```python
from build123d import *

# Parameters (mm, degrees)
SKETCH_W        = 76
SKETCH_H        = 22
PAD_DEPTH       = 76
SKETCH001_W     = 66
SKETCH001_H     = 26
PAD001_DEPTH    = 32
SKETCH002_W     = 62
SKETCH002_H     = 22
POCKET_DEPTH    = 30
SKETCH003_W     = 72
SKETCH003_H     = 18
POCKET001_DEPTH = 74
SKETCH004_W     = 30
SKETCH004_H     = 2
POCKET002_DEPTH = 30
SKETCH005_W     = 30
SKETCH005_H     = 2
POCKET003_DEPTH = 74


with BuildPart() as part:
    # Sketch → Pad (new body)
    with BuildSketch(Plane.XY):
        with Locations((38, 11)):
            Rectangle(SKETCH_W, SKETCH_H)
    extrude(amount=PAD_DEPTH)

    # Sketch001 → Pad001 (join)
    with BuildSketch(Plane.XY):
        with Locations((38, -13)):
            Rectangle(SKETCH001_W, SKETCH001_H)
    extrude(amount=PAD001_DEPTH)

    # Sketch002 (on Face4 of Pad001) → Pocket (cut)
    with BuildSketch(Plane.XY.offset(32)):
        with Locations((38, -13)):
            Rectangle(SKETCH002_W, SKETCH002_H)
    extrude(amount=-POCKET_DEPTH, mode=Mode.SUBTRACT)

    # Sketch003 (on Face7 of Pocket) → Pocket001 (cut)
    with BuildSketch(Plane.XY.offset(76)):
        with Locations((38, 11)):
            Rectangle(SKETCH003_W, SKETCH003_H)
    extrude(amount=-POCKET001_DEPTH, mode=Mode.SUBTRACT)

    # Sketch004 (on Face4 of Pocket001) → Pocket002 (cut)
    with BuildSketch(Plane.XY.offset(32)):
        with Locations((38, -1)):
            Rectangle(SKETCH004_W, SKETCH004_H)
    extrude(amount=-POCKET002_DEPTH, mode=Mode.SUBTRACT)

    # Sketch005 (on Face8 of Pocket002) → Pocket003 (cut)
    with BuildSketch(Plane.XY.offset(76)):
        with Locations((38, 1)):
            Rectangle(SKETCH005_W, SKETCH005_H)
    extrude(amount=-POCKET003_DEPTH, mode=Mode.SUBTRACT)


solid = part.part
```
Work out the finished part from the listing and answer in its coordinate system (mm). A direction names the side the tool comes from. Coordinates: 2 decimals unless noted, no trailing zeros. Write each loop counter-clockwise with the first axis right and the second up, starting at its lowest first coordinate (ties: lowest second). Pieces come first, ordered by that corner, then holes.
Q1. A cutting plane is placed at A-A, the plane z = 15. Give the vertices of the cut face in (x, y).
Q2. A cutting plane is placed at D-D, the plane z = 47. Give the vertices of the cut face in (x, y), then the cut area to 3 significant figures.
Q3. Which of the six approach directions +Z, -Z, +X, -X, +Y, -Y give full straight-line access (tool end or side, diameter ignored) to faces 4 (the face through (37, 20, 40)), 5 (the face through (71, -13, 16)), 6 (the face through (37.8, -24.5, 32)), 7 (the face through (5, -13, 16))?
Q4. Find the intervals of material crossed by line 1 (Y direction, x = 18, z = 24); line 2 (X direction, y = 12.5, z = 6.5); line 3 (Y direction, x = 20, z = 65.5), in increasing order.
Q5. Each of these flat-tipped pins is pushed along its axis until it touches: pin 1 Ø11 at (y, z) = (-18, 15) entering from +X; pin 2 Ø1 at (x, y) = (8.5, -9.5) entering from +Z; pin 3 Ø11.5 at (x, z) = (67, 55) entering from -Y. Where does it stop, or does it pass through?
Q6. A cutting plane is placed at C-C, the plane x = 51. Give the vertices of the cut face in (y, z), then the cut area to 3 significant figures.
Q7. A cutting plane is placed at B-B, the plane y = 12. Give the vertices of the cut face in (x, z), then the cut area to 3 significant figures.
Q8. Determine the mould class of faces 1 (the face through (37, 22, 37)), 2 (the face through (37, -2, 0)), 3 (the face through (2, 11, 40)) for opening direction Y: released by +Y, released by -Y, zero draft, split by the parting line, or undercut.
Findings below:
1. outline: (0, 0) - (5, 0) - (5, -26) - (71, -26) - (71, 0) - (76, 0) - (76, 22) - (0, 22) - close; hole (2, 2) - (23, 2) - (23, -2) - (7, -2) - (7, -24) - (69, -24) - (69, -2) - (53, -2) - (53, 2) - (74, 2) - (74, 20) - (2, 20) - close
2. outline: (0, 0) - (23, 0) - (23, 2) - (2, 2) - (2, 20) - (74, 20) - (74, 2) - (53, 2) - (53, 0) - (76, 0) - (76, 22) - (0, 22) - close
2. area: 316 mm2
3. face 4: +Z
3. face 5: +Z, -Z, +X, -Y
3. face 6: +Z, +X, -X, -Y
3. face 7: +Z, -Z, -X, -Y
4. line 1: y = -26 to -24, -2 to 2, 20 to 22
4. line 2: x = 0 to 2, 74 to 76
4. line 3: y = 0 to 2, 20 to 22
5. pin 1: stops at x = 71
5. pin 2: stops at z = 2
5. pin 3: stops at y = 0
6. outline: (-26, 0) - (22, 0) - (22, 76) - (20, 76) - (20, 2) - (-24, 2) - (-24, 32) - (-26, 32) - close
6. area: 304 mm2
7. outline: (0, 0) - (76, 0) - (76, 76) - (74, 76) - (74, 2) - (2, 2) - (2, 76) - (0, 76) - close
7. area: 448 mm2
8. face 1: released by +Y
8. face 2: zero draft
8. face 3: undercut
